from build123d import *

# Parameters (mm, degrees)
Y_KSEKLIK_EKSTR_ZYON1_DEPTH = 610
IZIM3_W                     = 10
IZIM3_H                     = 610
Y_KSEKLIK_EKSTR_ZYON2_DEPTH = 30
IZIM2_R                     = 35
KES_EKSTR_ZYON1_DEPTH       = 10


with BuildPart() as part:
    # Çizim1 → Yükseklik-Ekstrüzyon1 (new body)
    with BuildSketch(Plane.XY):
        Polygon((0, 0), (0, 200), (610, 200), (610, 0), (600, 0), (600, 190), (10, 190), (10, 0), align=None)
    extrude(amount=Y_KSEKLIK_EKSTR_ZYON1_DEPTH)

    # Çizim3 → Yükseklik-Ekstrüzyon2 (add)
    with BuildSketch(Plane.XZ):
        with Locations((5, 305)):
            Rectangle(IZIM3_W, IZIM3_H)
        with Locations((605, 305)):
            Rectangle(IZIM3_W, IZIM3_H)
    extrude(amount=Y_KSEKLIK_EKSTR_ZYON2_DEPTH)

    # Çizim2 → Kes-Ekstrüzyon1 (cut)
    with BuildSketch(Plane(origin=(0, 200, 0), x_dir=(1, 0, 0), z_dir=(0, 1, 0))):
        with Locations(Location((305, -305, 0), (0, 0, 270))):
            Circle(IZIM2_R)
        with BuildLine():
            ThreePointArc((305, -525), (460.563491861, -460.563491861), (525, -305))
            ThreePointArc((525, -305), (505, -285), (485, -305))
            ThreePointArc((485, -305), (432.279220614, -432.279220614), (305, -485))
            ThreePointArc((305, -485), (285, -505), (305, -525))
        make_face()
    extrude(amount=-KES_EKSTR_ZYON1_DEPTH, mode=Mode.SUBTRACT)


solid = part.part
Input: part model. Units: mm. Frame: model coordinates. A direction names the side the tool comes from. Give positions to 0.01 mm unless a question says otherwise; leave off trailing zeros. Order: outer loops, then holes, each group sorted by start corner. A loop starts at its lowest first (then second) coordinate and runs counter-clockwise, first axis right, second up. Notation, with made-up numbers: (83, -8.5) - (125, -8.5) arc R19 ccw to (125, 7.5) - close; hole circle Ø7 at (30, 89.5). An arc over 180 degrees is marked (long way). Answer as a JSON object with one key per item and string values. Group by question number.
Q1. Mould query, pull axis Z, two halves, no side actions, for faces 4 (the face through (285, 195, 505)), 5 (the face through (168, 196, 610)), 6 (the face through (10, 82, 301)). Classes: pulls with the +Z half, pulls with the -Z half, needs draft (parallel to the pull), parting line crosses it, or undercut.
Q2. Set-up query: faces 1 (the face through (600, 78, 301)), 2 (the face through (458.844, 195.07, 462.265)), 3 (the face through (610, 87, 301)). Return all of +Z, -Z, +X, -X, +Y, -Y with unobstructed straight access to the full face (end or side cutting, diameter ignored); none if empty.
Q3. Cut plane B-B, the plane x = 366.5. Output: boundary loops of the cut face in (y, z).
Q4. Cut plane C-C, the plane z = 425.5. Output: boundary loops of the cut face in (x, y).
Q5. Cut plane D-D, the plane z = 186.5. Output: boundary loops of the cut face in (x, y), then the cut area to 3 significant figures.
Q6. Line query: probe 1 along X at (y, z) = (196.5, 305); probe 2 along X at (y, z) = (37, 475); probe 3 along Y at (x, z) = (259, 94). Output: solid intervals per line, ascending.
Q7. Cut plane A-A, the plane y = 44.5. Output: boundary loops of the cut face in (x, z), then the cut area to 3 significant figures.
Q8. First-contact query: pin 1 Ø10 at (x, z) = (251.5, 242.5) entering from -Y. Flat tip, straight axial feed; report the tip coordinate or a pass-through.
Results:
{
 "1": {"face 4": "undercut", "face 5": "pulls with the +Z half", "face 6": "needs draft"},
 "2": {"face 1": "+Z, -Z, -Y", "face 2": "+Y, -Y", "face 3": "+Z, -Z, +X, +Y, -Y"},
 "3": {"outline": "(190, 0) - (200, 0) - (200, 474.17) - (190, 474.17) - close; (190, 516.23) - (200, 516.23) - (200, 610) - (190, 610) - close"},
 "4": {"outline": "(0, -30) - (10, -30) - (10, 190) - (438.72, 190) - (438.72, 200) - (0, 200) - close; (489.06, 190) - (600, 190) - (600, -30) - (610, -30) - (610, 200) - (489.06, 200) - close"},
 "5": {"outline": "(0, -30) - (10, -30) - (10, 190) - (600, 190) - (600, -30) - (610, -30) - (610, 200) - (0, 200) - close", "area": "10,500 mm^2"},
 "6": {"probe 1": "0 to 270, 340 to 485, 525 to 610", "probe 2": "0 to 10, 600 to 610", "probe 3": "190 to 200"},
 "7": {"outline": "(0, 0) - (10, 0) - (10, 610) - (0, 610) - close; (600, 0) - (610, 0) - (610, 610) - (600, 610) - close", "area": "12,200 mm^2"},
 "8": {"pin 1": "y = 190"}
}
